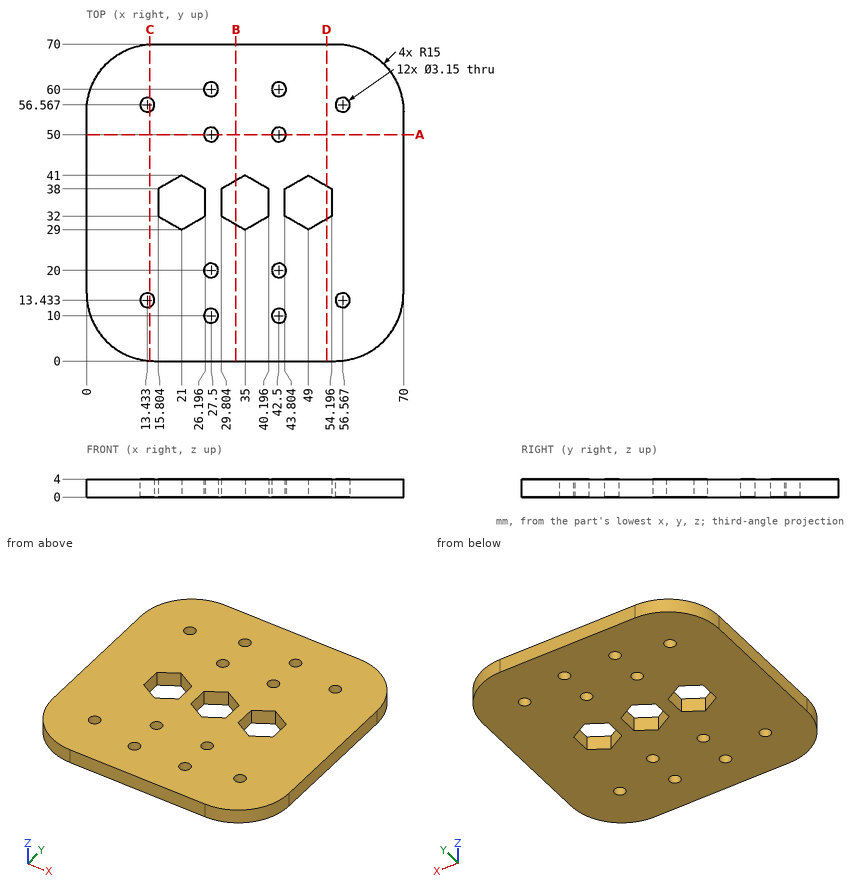
For this review, use the dimensioned drawing (mm, ordinates from the lowest corner) and the shaded views. Give positions to 0.01 mm unless a question says otherwise; leave off trailing zeros. Loops run counter-clockwise (first coordinate to the right, second up) from the corner with the lowest first, then second, coordinate; pieces in that order, holes last.
Item 1: For line 1 along X through (y, z) = (50, 2.5) (1 decimal); line 2 along X through (y, z) = (32.5, 0.3); line 3 along Y through (x, z) = (42.5, 3) (1 decimal), list the stretches that pass through material, from the lowest coordinate up.
Item 2: Take a section at A-A, the plane y = 50. State the section outline as (x, z) points (3 decimals).
Item 3: Insertion check: pin 1 (3 mm diameter, centred on x = 42.5, y = 60, fed in from -Z); pin 2 (2 mm diameter, centred on x = 10, z = 3.5, fed in from -Y). Each pin has a flat end and moves straight along its axis. Give the tip position at first contact, or say it passes through.
Item 4: Take a section at D-D, the plane x = 53. State the section outline as (y, z) points.
Item 5: Take a section at C-C, the plane x = 14. State the section outline as (y, z) points, and give its area (3 significant figures).
Item 6: Take a section at B-B, the plane x = 33. State the section outline as (y, z) points (1 decimal).
Calculated:
1. line 1: x = 0 to 25.9, 29.1 to 40.9, 44.1 to 70
1. line 2: x = 0 to 15.8, 26.2 to 29.8, 40.2 to 43.8, 54.2 to 70
1. line 3: y = 0 to 8.4, 11.6 to 18.4, 21.6 to 48.4, 51.6 to 58.4, 61.6 to 70
2. outline: (0, 0) - (25.925, 0) - (25.925, 4) - (0, 4) - close; (29.075, 0) - (40.925, 0) - (40.925, 4) - (29.075, 4) - close; (44.075, 0) - (70, 0) - (70, 4) - (44.075, 4) - close
3. pin 1: passes through
3. pin 2: stops at y = 0.54
4. outline: (0, 0) - (31.31, 0) - (31.31, 4) - (0, 4) - close; (38.69, 0) - (70, 0) - (70, 4) - (38.69, 4) - close
5. outline: (0.03, 0) - (11.96, 0) - (11.96, 4) - (0.03, 4) - close; (14.9, 0) - (55.1, 0) - (55.1, 4) - (14.9, 4) - close; (58.04, 0) - (69.97, 0) - (69.97, 4) - (58.04, 4) - close
5. area: 256 mm2
6. outline: (0, 0) - (30.2, 0) - (30.2, 4) - (0, 4) - close; (39.8, 0) - (70, 0) - (70, 4) - (39.8, 4) - close
